```python
from build123d import *

# Parameters (mm, degrees)
F0_R     = 13
F1_DEPTH = 3
F3_DEPTH = 3
F4_R     = 13
F4_R_2   = 10
F5_DEPTH = 9


with BuildPart() as f1:
    # F0 (on Top) → F1 (new body)
    with BuildSketch(Plane.XY):
        Circle(F0_R)
    extrude(amount=F1_DEPTH)

    # F2 (on face) → F3 (cut)
    with BuildSketch(Plane.XY.offset(3)):
        with BuildLine():
            Line((4.25, 4.25), (-4.25, 4.25))
            ThreePointArc((-4.25, 4.25), (-8.5, 0), (-4.25, -4.25))
            Line((-4.25, -4.25), (4.25, -4.25))
            ThreePointArc((4.25, -4.25), (8.5, 0), (4.25, 4.25))
        make_face()
    extrude(amount=-F3_DEPTH, mode=Mode.SUBTRACT)

    # F4 (on face) → F5 (join)
    with BuildSketch(Plane.XY.offset(3)):
        Circle(F4_R)
        Circle(F4_R_2, mode=Mode.SUBTRACT)
    extrude(amount=F5_DEPTH)


solid = f1.part
```
Here's how the part is built. I have some questions about the finished solid (model axes, mm). A direction names the side the tool comes from. Give positions to 0.01 mm unless a question says otherwise; leave off trailing zeros. Order: outer loops, then holes, each group sorted by start corner. A loop starts at its lowest first (then second) coordinate and runs counter-clockwise, first axis right, second up. Notation, with made-up numbers: M 55.25,62.25 L 72.25,62.25 A10 cw 72.25,70.25 Z; hole C -9,55 d6. An arc over 180 degrees is marked long. Use a Markdown table: item, result. Add a question column.
1. On a 3-axis mill with a long thin cutter (end or side, diameter ignored), from which of +Z, -Z, +X, -X, +Y, -Y can I reach the whole of each face in a straight line? I mean faces 1 (the flat face through (0, -6, 0)), 2 (the cylindrical face through (-2.17, -9.76, 7.44)), 3 (the flat face through (0, -4.25, 2)). Say none if no direction works.
2. Suppose I cut it at B-B (x = 0). List the corners of the cut face in (y, z) for me, and give its area (4 significant figures).
3. Suppose I cut it at C-C (z = 2). List the corners of the cut face in (x, y) for me.
4. If we mould it in two halves opening along X, with no side actions, what happens to faces 4 (the flat face through (0, 5, 3)), 5 (the flat face through (7, -8, 12)), 6 (the cylindrical face through (-10.316, -7.91, 5.916))? For each: +X half, -X half, draft (parallel to the pull), parting line (faces both ways), or undercut.
5. I need wall thicknesses on probe 1 along Y at (x, z) = (0, 6); probe 2 along Z at (x, y) = (-0.5, 9.75); probe 3 along Y at (x, z) = (-7.75, 1.25). Which ranges of each line are inside material? Lowest first, please. Write a range as from..to.
6. For pin 1 Ø1.5 at (x, y) = (-4, -3) entering from +Z; pin 2 Ø1 at (y, z) = (-5.5, 6.5) entering from +X; pin 3 Ø1.5 at (y, z) = (4.5, 3.5) entering from +X; pin 4 Ø6 at (x, y) = (0.5, -4) entering from +Z, each with a flat end and sliding along its axis, tell me the tip position at first contact or that it passes through.
7. Suppose I cut it at D-D (y = 5). List the corners of the cut face in (x, z) for me, and give its area (3 significant figures).
8. Suppose I cut it at A-A (y = 0). List the corners of the cut face in (x, z) for me.
Results list:
| question | item | result |
|---|---|---|
| 1 | face 1 | -Z, +X, -X, +Y, -Y |
| 1 | face 2 | +Z |
| 1 | face 3 | +Z, -Z |
| 2 | outline | M -13,0 L -4.25,0 L -4.25,3 L -10,3 L -10,12 L -13,12 Z; M 4.25,0 L 13,0 L 13,12 L 10,12 L 10,3 L 4.25,3 Z |
| 2 | area | 106.5 mm² |
| 3 | outline | C 0,0 d26; hole M -4.25,-4.25 L 4.25,-4.25 A4.25 ccw 4.25,4.25 L -4.25,4.25 A4.25 ccw Z |
| 4 | face 4 | undercut |
| 4 | face 5 | draft |
| 4 | face 6 | parting line |
| 5 | probe 1 | y = -13..-10, 10..13 |
| 5 | probe 2 | z = 0..3 |
| 5 | probe 3 | y = -10.44..-2.41, 2.41..10.44 |
| 6 | pin 1 | passes through |
| 6 | pin 2 | stops at x = 12 |
| 6 | pin 3 | stops at x = 12.45 |
| 6 | pin 4 | stops at z = 3 |
| 7 | outline | M -12,0 L 12,0 L 12,12 L 8.66,12 L 8.66,3 L -8.66,3 L -8.66,12 L -12,12 Z |
| 7 | area | 132 mm² |
| 8 | outline | M -13,0 L -8.5,0 L -8.5,3 L -10,3 L -10,12 L -13,12 Z; M 8.5,0 L 13,0 L 13,12 L 10,12 L 10,3 L 8.5,3 Z |
